Build history of the part. All positions in model axes, mm. A direction names the side the tool comes from. Give positions to 0.01 mm unless a question says otherwise; leave off trailing zeros. Loops run counter-clockwise (first coordinate to the right, second up) from the corner with the lowest first, then second, coordinate; pieces in that order, holes last. Notation, with made-up numbers: (38.5, 65) - (53.5, 65) arc R17 ccw to (53.5, 82) - close; hole circle Ø5 at (82, -32). An arc over 180 degrees is marked (long way). Return JSON: item names as keys, results as strings. Group by question number.
1) Drop a flat-ended pin along its axis: pin 1 (5 mm diameter, centred on x = -10.5, y = 38, fed in from -Z). Give the stop position or say it passes through.
2) Slice it at B-B (y = 32). List the corners of the cut face in (x, z), and give its area (3 significant figures).
3) Slice it at A-A (z = 1.15). List the corners of the cut face in (x, y).
4) Slice it at C-C (x = -25). List the corners of the cut face in (y, z).
5) Drill centre lines: probe 1 along Y at (x, z) = (-40, 1.8); probe 2 along X at (y, z) = (10.5, 0.8); probe 3 along Y at (x, z) = (-7.5, 0.5). Where is each one in solid material? Low to high. Write a range as from..to.
6) Mould opens along Y. For faces 3 (the face through (-13, 26, 2)), 4 (the face through (-40.45, 21.07, 0.99)), 5 (the face through (-43.51, 19.35, 0.99)) say: released by +Y, released by -Y, zero draft, split by the parting line, or undercut.
7) 3-axis set-ups, long thin cutter, end or side, ignore diameter. For faces 1 (the face through (-17.59, 13.49, 0.99)), 2 (the face through (-13, 26, 0)): which of +Z, -Z, +X, -X, +Y, -Y reach the whole face in a straight line?
```python
from build123d import *

# Parameters (mm, degrees)
SKETCH_1_R      = 1.5
EXTRUDE_1_DEPTH = 2


with BuildPart() as part:
    # 草圖1 → 填料-伸長1 (new body)
    with BuildSketch(Plane.XY):
        with BuildLine():
            ThreePointArc((-38.871013222, 17.001303806), (-17.306164288, 13.369084026), (0, 0))
            ThreePointArc((0, 0), (6.981013161, 17.661453415), (6.054619156, 36.629934525))
            ThreePointArc((6.054619156, 36.629934525), (-21.435485662, 41.318574281), (-43.626094088, 24.428751802))
            ThreePointArc((-43.626094088, 24.428751802), (-43.474451881, 19.289999171), (-38.871013222, 17.001303806))
        make_face()
        with Locations((-39.263484679, 21.985876622)):
            Circle(SKETCH_1_R, mode=Mode.SUBTRACT)
    extrude(amount=EXTRUDE_1_DEPTH)


solid = part.part
```
Results:
{
 "1": {"pin 1": "z = 0"},
 "2": {"outline": "(-37.91, 0) - (7.04, 0) - (7.04, 2) - (-37.91, 2) - close", "area": "89.9 mm2"},
 "3": {"outline": "(-43.63, 24.43) arc R5 ccw to (-38.87, 17) arc R45 cw to (0, 0) arc R45 ccw to (6.05, 36.63) arc R35 ccw to start; hole circle Ø3 at (-39.26, 21.99)"},
 "4": {"outline": "(15.94, 0) - (40.24, 0) - (40.24, 2) - (15.94, 2) - close"},
 "5": {"probe 1": "17.04..20.68, 23.29..29.71", "probe 2": "-11.81..5.18", "probe 3": "7.5..41.88"},
 "6": {"face 3": "zero draft", "face 4": "undercut", "face 5": "split by the parting line"},
 "7": {"face 1": "+Z, -Z, -Y", "face 2": "-Z, +X, -X, +Y, -Y"}
}
